Check sheet for the drawn part. Datum: minimum x, y, z corner. Units: mm. A direction names the side the tool comes from. Round coordinates to 2 decimals unless told otherwise and drop trailing zeros. Write each loop counter-clockwise with the first axis right and the second up, starting at its lowest first coordinate (ties: lowest second). Pieces come first, ordered by that corner, then holes. Notation, with made-up numbers: (16, -34.75) - (35, -34.75) arc R13 cw to (35, -18.75) - close; hole circle Ø1 at (63, -3). An arc over 180 degrees is marked (long way). Answer as a JSON object with one key per item and string values.
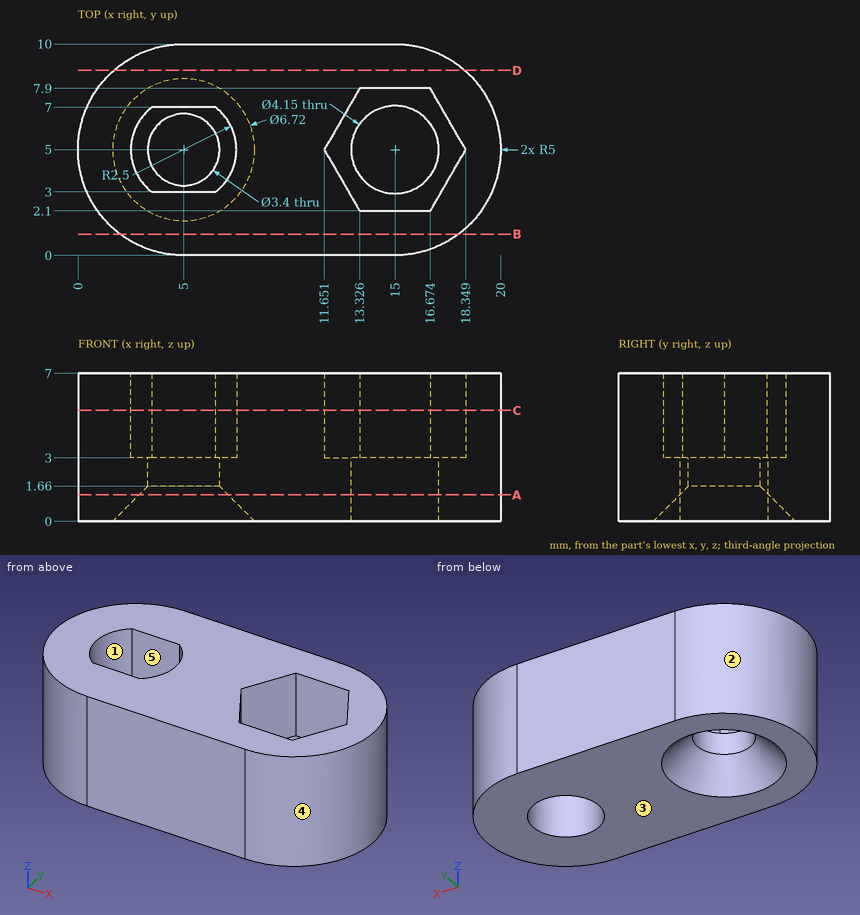
1. Cross-section at B-B (y = 1). Record the boundary of the cut face in (x, z), plus the area to 3 significant figures.
Completed:
{"outline": "(2, 0) - (18, 0) - (18, 7) - (2, 7) - close", "area": "112 mm^2"}
2. Access from +Z, -Z, +X, -X, +Y, -Y to the whole of each face (thin tool, end or side, straight path). Record for the marked faces 4 and 5.
Completed:
{"face 4": "+Z, -Z, +X", "face 5": "+Z"}
3. Cross-section at D-D (y = 8.75). Record the boundary of the cut face in (x, z), plus the area to 3 significant figures.
Completed:
{"outline": "(1.69, 0) - (18.31, 0) - (18.31, 7) - (1.69, 7) - close", "area": "116 mm^2"}
4. Cross-section at C-C (z = 5.25). Record the boundary of the cut face in (x, y) (1 decimal).
Completed:
{"outline": "(5, 0) - (15, 0) arc R5 ccw to (15, 10) - (5, 10) arc R5 ccw to start; hole (3.5, 3) - (6.5, 3) arc R2.5 ccw to (6.5, 7) - (3.5, 7) arc R2.5 ccw to start; hole (11.7, 5) - (13.3, 2.1) - (16.7, 2.1) - (18.3, 5) - (16.7, 7.9) - (13.3, 7.9) - close"}
5. Material ranges on probe 1 along Y at (x, z) = (5, 2.45); probe 2 along Y at (x, z) = (15, 1.2) (1 decimal); probe 3 along Z at (x, y) = (17.5, 4.75), recorded low to high. Write a range as from..to.
Completed:
{"probe 1": "y = 0..3.3, 6.7..10", "probe 2": "y = 0..2.9, 7.1..10", "probe 3": "z = 0..3"}
6. Go/stop test with flat-tipped pins: pin 1 (3.5 mm diameter, centred on x = 15, y = 5, fed in from +Z); pin 2 (4 mm diameter, centred on y = 8, z = 3, fed in from -X); pin 3 (3 mm diameter, centred on x = 16.5, z = 4.5, fed in from +Y); pin 4 (1 mm diameter, centred on x = 3.5, y = 5.5, fed in from -Z). Record where each tip stops, or that it passes through.
Completed:
{"pin 1": "passes through", "pin 2": "stops at x = 0.1", "pin 3": "stops at y = 10", "pin 4": "stops at z = 1.28"}
7. Cross-section at A-A (z = 1.25). Count the separate pieces of the cut face and the enclosed holes in it, plus the area to 3 significant figures.
Completed:
{"separate pieces": "1", "enclosed holes": "2", "area": "151 mm^2"}
8. Mould release check, pull along Y, two halves, no side actions. Record for the marked faces 1, 2 and 3: released by +Y, released by -Y, zero draft, split by the parting line, or undercut.
Completed:
{"face 1": "undercut", "face 2": "split by the parting line", "face 3": "zero draft"}
